Input: part model. Units: mm. Frame: model coordinates. A direction names the side the tool comes from. Coordinates: 2 decimals unless noted, no trailing zeros. Loops run counter-clockwise (first coordinate to the right, second up) from the corner with the lowest first, then second, coordinate; pieces in that order, holes last. Notation, with made-up numbers: (56.25, -39.75) -> (107.25, -39.75) arc R26 ccw to (107.25, -10.75) -> close; hole circle Ø3 at (83.25, 69.5). An arc over 180 degrees is marked (long way). Answer as a JSON object with one key per item and string values.
from build123d import *

# Parameters (mm, degrees)
SKETCH_1_R          = 7.75
SKETCH_1_R_2        = 1.25
SKETCH_1_R_3        = 1.65
SKETCH_1_R_4        = 1.75
SKETCH_1_W          = 5.081480492
SKETCH_1_H          = 8.790007362
EXTRUDE_1_DEPTH     = 4.5
SKETCH_2_R          = 8.5
CUT_EXTRUDE_1_DEPTH = 0.8
FILLET_1_R          = 4
CUT_EXTRUDE_2_DEPTH = 2


with BuildPart() as part:
    # 草图1 → 凸台-拉伸1 (new body)
    with BuildSketch(Plane.XY):
        with BuildLine():
            Line((-10, 0), (-10, -12.123829059))
            Line((-10, -12.123829059), (-5.144235045, -15.224714909))
            Line((-5.144235045, -15.224714909), (-3.96721445, -30.511086595))
            ThreePointArc((-3.96721445, -30.511086595), (0, -34), (3.96721445, -30.511086595))
            Line((3.96721445, -30.511086595), (5.144235045, -15.224714909))
            Line((5.144235045, -15.224714909), (10, -12.123829059))
            Line((10, -12.123829059), (10, 0))
            ThreePointArc((10, 0), (0, 10), (-10, 0))
        make_face()
        Circle(SKETCH_1_R, mode=Mode.SUBTRACT)
        with Locations((-7, -9.124143795)):
            Circle(SKETCH_1_R_2, mode=Mode.SUBTRACT)
        with Locations((7, -9.124143795)):
            Circle(SKETCH_1_R_2, mode=Mode.SUBTRACT)
        with Locations((0, -30)):
            Circle(SKETCH_1_R_3, mode=Mode.SUBTRACT)
        with Locations((0, -24)):
            Circle(SKETCH_1_R_4, mode=Mode.SUBTRACT)
        with Locations((0, -15.224714909)):
            Rectangle(SKETCH_1_W, SKETCH_1_H, mode=Mode.SUBTRACT)
    extrude(amount=EXTRUDE_1_DEPTH)

    # 草图2 → 切除-拉伸1 (cut)
    with BuildSketch(Plane.XY.offset(4.5)):
        Circle(SKETCH_2_R)
    extrude(amount=-CUT_EXTRUDE_1_DEPTH, mode=Mode.SUBTRACT)

    # 圆角1
    fillet_1_edges = [part.edges().sort_by_distance(p)[0] for p in [
        (-5.144235045, -15.224714909, 2.25),
        (-10, -12.123829059, 2.25),
        (10, -12.123829059, 2.25),
        (5.144235045, -15.224714909, 2.25),
    ]]
    fillet(fillet_1_edges, radius=FILLET_1_R)

    # 草图3 → 切除-拉伸2 (cut)
    with BuildSketch(Plane.XY.offset(4.5)):
        Polygon((7, -6.641537638), (9.15, -7.882840717), (9.15, -10.365446874), (7, -11.606749953), (4.85, -10.365446874), (4.85, -7.882840717), align=None)
        Polygon((-7, -6.641537638), (-4.85, -7.882840717), (-4.85, -10.365446874), (-7, -11.606749953), (-9.15, -10.365446874), (-9.15, -7.882840717), align=None)
    extrude(amount=-CUT_EXTRUDE_2_DEPTH, mode=Mode.SUBTRACT)


solid = part.part
1. Section query C-C (z = 0.9). Return loops of the section in (x, y).
Reply:
{"outline": "(-10, -9.93) arc R4 ccw to (-8.15, -13.3) -> (-6.83, -14.15) arc R4 cw to (-4.99, -17.21) -> (-3.97, -30.51) arc R4 ccw to (3.97, -30.51) -> (4.99, -17.21) arc R4 cw to (6.83, -14.15) -> (8.15, -13.3) arc R4 ccw to (10, -9.93) -> (10, 0) arc R10 ccw to (-10, 0) -> close; hole circle Ø2.5 at (-7, -9.12); hole circle Ø15.5 at (0, 0); hole (-2.54, -19.62) -> (2.54, -19.62) -> (2.54, -10.83) -> (-2.54, -10.83) -> close; hole circle Ø3.5 at (0, -24); hole circle Ø3.3 at (0, -30); hole circle Ø2.5 at (7, -9.12)"}
2. Pin query (flat end, axial travel): P1, Ø2, axis at x = -7, y = -9.12, coming from the -Z side; P2, Ø2, axis at x = 7, y = -10, coming from the +Z side; P3, Ø1, axis at y = -27.5, z = 3.5, coming from the +X side; P4, Ø1, axis at x = -7, z = 3.5, coming from the -Y side. Return the tip coordinate at first contact, or that it passes through.
Reply:
{"P1": "passes through", "P2": "stops at z = 2.5", "P3": "stops at x = 4.24", "P4": "stops at y = -14.38"}
3. Section query B-B (y = 0.5). Return loops of the section in (x, z).
Reply:
{"outline": "(-9.99, 0) -> (-7.73, 0) -> (-7.73, 3.7) -> (-8.49, 3.7) -> (-8.49, 4.5) -> (-9.99, 4.5) -> close; (7.73, 0) -> (9.99, 0) -> (9.99, 4.5) -> (8.49, 4.5) -> (8.49, 3.7) -> (7.73, 3.7) -> close"}
4. Section query D-D (y = -27.5). Return loops of the section in (x, z), plus the area to 3 significant figures.
Reply:
{"outline": "(-4.2, 0) -> (4.2, 0) -> (4.2, 4.5) -> (-4.2, 4.5) -> close", "area": "37.8 mm2"}
5. Access query for faces 1 (the face through (5.94, -10.995, 3.514)), 2 (the face through (0, -19.62, 2)), 3 (the face through (-2, -10, 4.5)). Directions: +Z, -Z, +X, -X, +Y, -Y. A direction counts if a zero-diameter tool reaches every point of the face in a straight line with its end or side. Return the directions, or none.
Reply:
{"face 1": "+Z", "face 2": "+Z, -Z", "face 3": "+Z, +X, -X, +Y, -Y"}
6. Section query A-A (x = 0). Return loops of the section in (y, z).
Reply:
{"outline": "(-34, 0) -> (-31.65, 0) -> (-31.65, 4.5) -> (-34, 4.5) -> close; (-28.35, 0) -> (-25.75, 0) -> (-25.75, 4.5) -> (-28.35, 4.5) -> close; (-22.25, 0) -> (-19.62, 0) -> (-19.62, 4.5) -> (-22.25, 4.5) -> close; (-10.83, 0) -> (-7.75, 0) -> (-7.75, 3.7) -> (-8.5, 3.7) -> (-8.5, 4.5) -> (-10.83, 4.5) -> close; (7.75, 0) -> (10, 0) -> (10, 4.5) -> (8.5, 4.5) -> (8.5, 3.7) -> (7.75, 3.7) -> close"}
7. Line query: line 1 along X through (y, z) = (-10, 4.25); line 2 along Y through (x, z) = (7, 1.6); line 3 along Y through (x, z) = (0.25, 1). Output: solid intervals per line, ascending.
Reply:
{"line 1": "x = -10 to -9.15, -4.85 to 4.85, 9.15 to 10", "line 2": "y = -14.04 to -10.37, -7.87 to -3.33, 3.33 to 7.14", "line 3": "y = -33.99 to -31.63, -28.37 to -25.73, -22.27 to -19.62, -10.83 to -7.75, 7.75 to 10"}
8. Mould query, pull axis Y, two halves, no side actions, for faces 4 (the face through (-4.486, -23.77, 2.218)), 5 (the face through (5.91, -7.27, 3.51)), 6 (the face through (0, 10, 2)), 7 (the face through (4.85, -9, 4)). Classes: pulls with the +Y half, pulls with the -Y half, needs draft (parallel to the pull), parting line crosses it, or undercut.
Reply:
{"face 4": "pulls with the -Y half", "face 5": "undercut", "face 6": "pulls with the +Y half", "face 7": "undercut"}
